from build123d import *

# Parameters (mm, degrees)
SKETCH1_W                                      = 5
SKETCH1_H                                      = 60
EXTRUDE_THIN1_DEPTH                            = 100
SKETCH3_R                                      = 5
SKETCH13_R                                     = 3.5
CUT_EXTRUDE1_DEPTH                             = 211.535032714
CSK_FOR_M8_FLAT_HEAD_MACHINE_SCREW1_AT_2_COUNT = 2
CSK_FOR_M8_FLAT_HEAD_MACHINE_SCREW1_AT_2_PITCH = 53.800041305
F_2CUTS_DEPTH                                  = 120.373363863
F_2CUTS_DEPTH_BACK                             = 120.373363863
SKETCH23_W                                     = 42
SKETCH23_H                                     = 11


with BuildPart() as part:
    # Sketch1 → Extrude-Thin1 (new, symmetric)
    with BuildSketch(Plane.XY):
        with Locations((2.5, 30)):
            Rectangle(SKETCH1_W, SKETCH1_H)
    extrude(amount=EXTRUDE_THIN1_DEPTH, both=True)

    # Sweep5: sweep along a curve in space
    with BuildLine() as sweep5_path:
        Line((5, 60, 100), (5, 60, -100))
    # Sketch3 → Sweep5 (sweep)
    with BuildSketch(Plane.XY.offset(100)):
        with Locations((5, 60)):
            Circle(SKETCH3_R)
    sweep(path=sweep5_path.line)

    # Sketch13 → Cut-Extrude1 (cut, through all)
    with BuildSketch(Plane.XY.offset(100)):
        with Locations((5, 60)):
            Circle(SKETCH13_R)
    extrude(amount=-CUT_EXTRUDE1_DEPTH, mode=Mode.SUBTRACT)

    # Sketch15 → CSK for M8 Flat Head Machine Screw1 (revolve, cut)
    with BuildSketch(Plane(origin=(5, 30, 85), x_dir=(0, 0, -1), z_dir=(0, 1, 0))):
        Polygon((0, 0), (0, 5), (4.5, 5), (4.5, 4.15), (8.65, 0), align=None)
    csk_for_m8_flat_head_machine_screw1 = revolve(axis=Axis((11.35, 30, 85), (-1, 0, 0)), mode=Mode.SUBTRACT)

    # CSK for M8 Flat Head Machine Screw1 at 2: CSK for M8 Flat Head Machine Screw1 ×2
    with Locations(*[Vector(0, -0.2788101948639555, -0.9603462267536241) * (i * CSK_FOR_M8_FLAT_HEAD_MACHINE_SCREW1_AT_2_PITCH) for i in range(1, CSK_FOR_M8_FLAT_HEAD_MACHINE_SCREW1_AT_2_COUNT)]):
        add(csk_for_m8_flat_head_machine_screw1, mode=Mode.SUBTRACT)

    # Mirror1: CSK for M8 Flat Head Machine Screw1 across plane
    add(csk_for_m8_flat_head_machine_screw1.mirror(Plane.XY), mode=Mode.SUBTRACT)

    # Mirror1 copy 1 sketch → Mirror1 copy 1 (revolve, cut)
    with BuildSketch(Plane(origin=(5, 15, -33.333333333), x_dir=(0, 0, 1), z_dir=(0, 1, 0))):
        Polygon((0, 0), (0, -5), (4.5, -5), (4.5, -4.15), (8.65, 0), align=None)
    revolve(axis=Axis((11.35, 15, -33.333333333), (1, 0, 0)), mode=Mode.SUBTRACT)

    # Sketch23 → 2Cuts (cut, two sides: drawn at the far end of the back side and taken through both)
    with BuildSketch(Plane(origin=(5, 0, 0), x_dir=(0, 0, -1), z_dir=(1, 0, 0)).offset(-F_2CUTS_DEPTH_BACK)):
        with Locations((-40, 59.5)):
            Rectangle(SKETCH23_W, SKETCH23_H)
        with Locations((40, 59.5)):
            Rectangle(SKETCH23_W, SKETCH23_H)
    extrude(amount=F_2CUTS_DEPTH + F_2CUTS_DEPTH_BACK, mode=Mode.SUBTRACT)


solid = part.part
Source: CAD feature listing. Evaluate the final solid. Frame: model axes, mm. A direction names the side the tool comes from. Coordinates: 2 decimals unless noted, no trailing zeros. Loops run counter-clockwise (first coordinate to the right, second up) from the corner with the lowest first, then second, coordinate; pieces in that order, holes last. Notation, with made-up numbers: M 19.5,-38 L 69.5,-38 A33 cw 69.5,-3 Z; hole C 15.25,49 d6. An arc over 180 degrees is marked long. Answer in a Markdown table with one row per item.
Q1. Section C-C on z = 46. Return the cut outline in (x, y).
Answers below:
| item | result |
|---|---|
| outline | M 0,0 L 5,0 L 5,54 L 0,54 Z |
Q2. Ray query, probe 1 along Z at (x, y) = (0.55, 30); probe 2 along Z at (x, y) = (3, 35); probe 3 along X at (y, z) = (33.5, -56.5). Return the intervals inside material, ascending. Write a range as from..to.
Answers below:
| item | result |
|---|---|
| probe 1 | z = -100..-89.5, -80.5..80.5, 89.5..100 |
| probe 2 | z = -100..-89.38, -80.62..80.62, 89.38..100 |
| probe 3 | x = 0..5 |
Q3. Draft query along Z for faces 3 (the conical face through (1.11, 26.783, 88.508)), 4 (the cylindrical face through (8.34, 61.05, -80.23)), 5 (the flat face through (3, 33, -100)). Return one class per face: pulls with the +Z half, pulls with the -Z half, needs draft (parallel to the pull), parting line crosses it, or undercut.
Answers below:
| item | result |
|---|---|
| face 3 | undercut |
| face 4 | needs draft |
| face 5 | pulls with the -Z half |
Q4. Section A-A on z = 85. Return the cut outline in (x, y).
Answers below:
| item | result |
|---|---|
| outline | M 0,0 L 5,0 L 5,21.35 L 0.85,25.5 L 0,25.5 Z; M 0,34.5 L 0.85,34.5 L 5,38.65 L 5,55 A5 ccw long 0,60 Z; hole C 5,60 d7 |
Q5. Section B-B on z = -15.5. Return the cut outline in (x, y), plus the area to 3 significant figures.
Answers below:
| item | result |
|---|---|
| outline | M 0,0 L 5,0 L 5,55 A5 ccw long 0,60 Z; hole C 5,60 d7 |
| area | 320 mm^2 |
Q6. First-contact query: pin 1 (5 mm diameter, centred on x = 5, y = 61.5, fed in from -Z); pin 2 (1 mm diameter, centred on y = 40.5, z = 74, fed in from +X); pin 3 (2.5 mm diameter, centred on x = 3.5, z = -47.5, fed in from +Y). Flat tips, straight axial feed; report the tip coordinate or a pass-through.
Answers below:
| item | result |
|---|---|
| pin 1 | stops at z = -100 |
| pin 2 | stops at x = 5 |
| pin 3 | stops at y = 54 |
Q7. Set-up query: faces 1 (the flat face through (2.7, 57, 19)), 2 (the conical face through (1.11, 19.223, -31.137)). Return all of +Z, -Z, +X, -X, +Y, -Y with unobstructed straight access to the full face (end or side cutting, diameter ignored); none if empty.
Answers below:
| item | result |
|---|---|
| face 1 | +X, -X, +Y |
| face 2 | +X |
